Here's how the part is built. I have some questions about the finished solid (model axes, mm). Face numbers are marked on the shaded views. A direction names the side the tool comes from. Give positions to 0.01 mm unless a question says otherwise; leave off trailing zeros. Loops run counter-clockwise (first coordinate to the right, second up) from the corner with the lowest first, then second, coordinate; pieces in that order, holes last.
Q1. I need wall thicknesses on line 1 (Y direction, x = -2, z = -0.8); line 2 (X direction, y = 2, z = -1.55); line 3 (X direction, y = 12, z = -2.4). Which ranges of each line are inside material? Lowest first, please.
Q2. If we section it at A-A (x = 21.5): Please give me the cut outline in (y, z), plus the area to 3 significant figures.
Q3. We'd pull the mould along X, two halves only. Please class the marked faces 1, 2, 3 and 4: +X half, -X half, draft (parallel to the pull), parting line (faces both ways), or undercut.
Q4. If we section it at C-C (x = -9): Give the number of separate pieces and of enclosed holes in the cut face, plus the area to 3 significant figures.
Q5. If we section it at B-B (y = 1.5): Please give me the cut outline in (x, z).
Q6. For the marked faces 5 and 6, which set-ups out of +Z, -Z, +X, -X, +Y, -Y let a thin tool reach every point of the face, with its end or its side?
Q7. Will these pins go through, and if not, where does the flat tip stop? P1, Ø4, axis at x = 14.5, y = 3, coming from the -Z side; P2, Ø1, axis at y = 1.5, z = -2.5, coming from the +X side; P3, Ø1, axis at y = -2.5, z = -2, coming from the +X side.
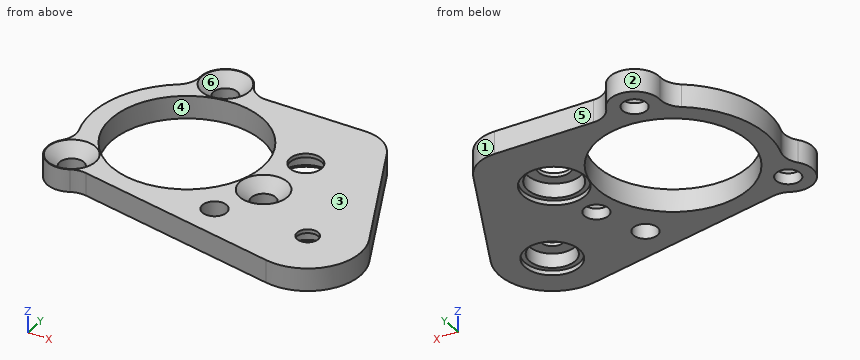
Autodesk Inventor part; units mm, degrees
ref_plane "YZ Plane" through (0, 0, 0) normal (1, 0, 0) x (0, 1, 0)
ref_plane "XZ Plane" through (0, 0, 0) normal (0, 1, 0) x (-1, 0, 0)
ref_plane "XY Plane" through (0, 0, 0) normal (0, 0, 1) x (1, 0, 0)
sketch "Sketch1" plane through (0, 0, 0) normal (0, 0, 1) x (1, 0, 0)
  circle A0 centre (0, 0) radius 10
  circle A1 centre (0, 0) radius 12.5
  circle A2 centre (0, 0) radius 4.9 construction
  circle A3 centre (0, 0) radius 2.6
  circle A4 centre (22, -10) radius 6.25 construction
  circle A5 centre (13.7949, 3.1501) radius 9.25 construction
  circle A6 centre (22, -10) radius 7
  circle A7 centre (10, -10.5) radius 1.6
  circle A8 centre (10, -10.5) radius 3.75
  line L0 (-7.6132, -11.2269) -> (20.6297, -16.8646)
  line L1 (0, 12.5) -> (16.0464, 12.5)
  line L2 (20.5779, 9.6131) -> (28.3442, -7.0417)
  arc A9 (20.5779, 9.6131) -> (16.0464, 12.5) centre (16.0464, 7.5) ccw
  circle A10 centre (13.7949, 3.1501) radius 2.1
  circle A11 centre (13.7949, 3.1501) radius 3.5125
  circle A12 centre (13.7949, 3.1501) radius 4.1125
  circle A13 centre (22, -10) radius 1.4
  circle A14 centre (22, -10) radius 3.0125
  circle A15 centre (22, -10) radius 3.6125
  circle A16 centre (-9.8467, -8.866) radius 3.25
  circle A17 centre (-9.8467, -8.866) radius 1.6
  circle A18 centre (12.6015, -4.0945) radius 3.25
  circle A19 centre (12.6015, -4.0945) radius 1.6
  circle A20 centre (-2.7548, 12.9605) radius 3.25
  circle A21 centre (-2.7548, 12.9605) radius 1.6
  line L3 (0, 0) -> (-9.2893, -8.3641) construction
  line L4 (0, 0) -> (12.5, 0) construction
  arc A22 (9.6868, -12.069) -> (10.3132, -8.931) centre (10, -10.5) ccw
  point P0 (-2.4469, -12.2582)
  point P1 (0.4624, 12.5)
  point P2 (-5.502, 11.224)
  point P3 (-11.0485, -5.8464)
  point P4 (-6.9692, -10.3769)
  dimension "d33" = 6.5
  dimension "d0" = 20
  dimension "d1" = 25
  dimension "d2" = 9.8
  dimension "d3" = 5.2
  dimension "d4" = 22
  dimension "d5" = 10
  dimension "d6" = 12.5
  dimension "d7" = 18.5
  dimension "d8" = 14
  dimension "d9" = 3.2
  dimension "d10" = 10.5
  dimension "d11" = 10
  dimension "d12" = 7.5
  dimension "d13" = 115
  dimension "d14" = 5
  dimension "d15" = 4.2
  dimension "d16" = 7.025
  dimension "d17" = 8.225
  dimension "d18" = 2.8
  dimension "d19" = 6.025
  dimension "d20" = 7.225
  dimension "d34" = 3.2
  dimension "d37" = 360
  dimension "d39" = 12.5
  dimension "d40" = 138
extrude "Extrusion1" add sketch "Sketch1" against normal blind 3 contours A0 A20 A1 A12 A18 | A0 A16 A1 A20 | A20 A1 A21 | A18 A1 A8 A16 A0 | A18 A1 A19 | A16 A1 A17 | A20 L1 A1 A21 | A20 L1 A9 L2 A6 L0 A1 A8 A18 A12 | A1 L1 A20 | A18 A12 A8 A1 A19 | A1 A12 A18 | A18 A8 A1 | A1 A17 A16 | A21 A1 | A1 A21 | A12 A18 A1 A11 | A1 A11 A12 | A19 A1 | A1 A19 | A18 A12 | A8 A18 A1 | A1 A8 | A8 A18 | A1 L0 A16 | A17 A1 | A1 A17 | A11 A1 A10 | A1 A10 A11 | A6 | A14 | A15
extrude "Extrusion2" cut sketch "Sketch1" along normal blind 0.6 from surface at -3 contours A12 A18 A1 A11 | A1 A11 A12 | A18 A12 | A15
extrude "Extrusion3" cut sketch "Sketch1" along normal blind 2.5 from surface at -3 contours A11 A1 A10 | A1 A10 A11 | A14
fillet "Fillet1" radius 3 4 edges at (-11.0485, -5.8464, -1.5) (-5.502, 11.224, -1.5) (0.4624, 12.5, -1.5) (-7.6132, -11.2269, -1.5)
hole "Hole1" at (-2.7548, 12.9605, 0) at (-9.8467, -8.866, 0) at (12.6015, -4.0945, 0) direction (0, 0, -1) diameter 3.2 depth 6 countersink diameter 6.3 countersink angle 90
properties part number "Dribbler Bracket A"
Check sheet entries:
1. line 1: y = -12.35 to -9.8, 9.8 to 10.74, 15.19 to 16.12
1. line 2: x = -12.34 to -9.8, 9.8 to 10.48, 17.11 to 24.13
1. line 3: x = -6.06 to -4.03, -1.48 to 18.23
2. outline: (-16.98, -3) - (-13.58, -3) - (-13.58, -2.4) - (-12.97, -2.4) - (-12.97, -0.5) - (-11.31, -0.5) - (-11.31, 0) - (-16.98, 0) - close; (-8.69, -0.5) - (-7.03, -0.5) - (-7.03, -2.4) - (-6.42, -2.4) - (-6.42, -3) - (7.64, -3) - (7.64, 0) - (-8.69, 0) - close
2. area: 57.0 mm2
3. face 1: +X half
3. face 2: parting line
3. face 3: draft
3. face 4: undercut
4. separate pieces: 3
4. enclosed holes: 0
4. area: 25.1 mm2
5. outline: (-12.41, -3) - (-9.89, -3) - (-9.89, 0) - (-12.41, 0) - close; (9.89, -3) - (10.03, -3) - (10.03, -2.4) - (10.69, -2.4) - (10.69, -0.5) - (12.5, -0.5) - (12.5, 0) - (9.89, 0) - close; (15.09, -0.5) - (16.9, -0.5) - (16.9, -2.4) - (17.56, -2.4) - (17.56, -3) - (24.36, -3) - (24.36, 0) - (15.09, 0) - close
6. face 5: +Z, -Z, +X, +Y
6. face 6: +Z
7. P1: stops at z = -0.5
7. P2: stops at x = 24.59
7. P3: stops at x = 26.46
